Geometry: final body of the model. Coordinates: model frame, mm. A direction names the side the tool comes from. Give positions to 0.01 mm unless a question says otherwise; leave off trailing zeros.
Q1. Reachability of faces 1 (the cylindrical face through (66.487, 109.322, -2.748)), 2 (the cylindrical face through (-97.114, -89.051, 9.903)), 3 (the cylindrical face through (40.74, -98.25, 4.38)) from +Z, -Z, +X, -X, +Y, -Y: full face, straight path, thin tool, end or side. Return the list, or none.
Q2. Pin query (flat end, axial travel): pin 1 Ø3.5 at (x, y) = (63.5, -109.99) entering from -Z; pin 2 Ø1.5 at (y, z) = (26, -4) entering from -X; pin 3 Ø5 at (x, y) = (63.5, 109.99) entering from +Z; pin 4 Ø7 at (x, y) = (-63.5, 109.99) entering from -Z. Return the tip coordinate at first contact, or that it passes through.
Q3. Line query: line 1 (X direction, y = -3.5, z = 8); line 2 (X direction, y = 0, z = 4.25); line 3 (Y direction, x = -63.5, z = -3.5). Output: solid intervals per line, ascending.
Autodesk Inventor part; units mm, degrees
ref_plane "YZ Plane" through (0, 0, 0) normal (1, 0, 0) x (0, 1, 0)
ref_plane "XZ Plane" through (0, 0, 0) normal (0, 1, 0) x (-1, 0, 0)
ref_plane "XY Plane" through (0, 0, 0) normal (0, 0, 1) x (1, 0, 0)
sketch "Sketch1" plane through (0, 0, 0) normal (1, 0, 0) x (0, 1, 0)
  arc A0 (-107.5189, 2.6268) -> (-107.5189, -2.6268) centre (-105.3147, 0) ccw
  line L0 (-105.5687, 3.175) -> (-105.5687, -3.175) construction
  line L1 (-107.5189, 2.6268) -> (-107.5189, 4.635) construction
  line L2 (-106.3625, 5.1846) -> (-106.3625, 3.5971)
  line L3 (-107.5189, 2.6268) -> (-106.3625, 3.5971)
  line L4 (-107.5189, -2.6268) -> (-106.3625, -3.5971)
  line L5 (-134.9375, 5.1846) -> (-134.9375, -6.7721)
  line L6 (-134.9375, 5.1846) -> (-106.3625, 5.1846)
  line L7 (-134.9375, -6.7721) -> (-106.3625, -6.7721)
  line L8 (-106.3625, -6.7721) -> (-106.3625, -3.5971)
  circle A1 centre (-105.5687, 0) radius 3.175 construction
  line L9 (-35.1032, 0) -> (87.3968, 0) construction
  line L10 (-104.775, 5.1846) -> (-104.775, 3.5971) construction
  line L11 (-104.775, -6.7721) -> (-104.775, -3.5971) construction
  line L12 (-103.6186, 2.6268) -> (-104.775, 3.5971) construction
  line L13 (-103.6186, -2.6268) -> (-104.775, -3.5971) construction
  arc A2 (-103.6186, -2.6268) -> (-103.6186, 2.6268) centre (-105.8227, 0) ccw construction
  line L14 (-79.375, 5.1846) -> (-79.375, -6.7721) construction
  line L15 (0, -7.2584) -> (0, 7.2584) construction
  line L16 (-79.375, -6.7721) -> (-104.775, -6.7721) construction
  line L17 (-79.375, 5.1846) -> (-104.775, 5.1846) construction
  line L18 (-104.775, 5.1846) -> (-104.775, 8.3596) construction
  line L19 (-104.775, 8.3596) -> (-79.375, 8.3596) construction
  line L20 (-79.375, 8.3596) -> (-79.375, 5.1846) construction
  line L21 (-90.4875, 22.7342) -> (-90.4875, 8.3596) construction
  point P0 (0, 0)
  point P1 (0, 0)
  point P2 (-108.7437, 0)
  point P3 (-134.9375, -0.7938)
  point P4 (-19.1031, 0)
  point P5 (0, 7.2584)
  point P6 (0, 0)
  point P7 (-119.9381, 21.0485)
  dimension "d0" = 6.35
  dimension "d1" = 3.429
  dimension "d2" = 50
  dimension "d3" = 3.175
  dimension "d4" = 1.5875
  dimension "d5" = 158.75
  dimension "d6" = 3.175
  dimension "d7" = 25.4
  dimension "d8" = 28.575
  dimension "d9" = 180.975
  dimension "d31" = 1.5875
revolve "Revolution1" add sketch "Sketch1" angle 360 about axis through (0, 0, -7.2584) along (0, 0, 1)
sketch "Sketch2" plane through (0, 0, -6.7721) normal (0, 0, 1) x (1, 0, 0)
  point P0 (0, 0)
  point P1 (-127, 0)
  point P2 (-109.9852, -63.5)
  point P3 (-63.5, -109.9852)
  point P4 (0, -127)
  point P5 (63.5, -109.9852)
  point P6 (109.9852, -63.5)
  point P7 (127, 0)
  point P8 (109.9852, 63.5)
  point P9 (63.5, 109.9852)
  point P10 (0, 127)
  point P11 (-63.5, 109.9852)
  point P12 (-109.9852, 63.5)
  dimension "d11" = 127
  dimension "d14" = 360
hole "Hole1" at (-109.9852, -63.5, -6.7721) at (-63.5, -109.9852, -6.7721) at (63.5, -109.9852, -6.7721) at (109.9852, -63.5, -6.7721) at (109.9852, 63.5, -6.7721) at (63.5, 109.9852, -6.7721) at (-63.5, 109.9852, -6.7721) at (-109.9852, 63.5, -6.7721) direction (0, 0, 1) diameter 6.12 depth 7.9375 tip angle 118
sketch "Sketch3" plane through (0, 0, 5.1846) normal (0, 0, 1) x (1, 0, 0)
  circle A0 centre (0, 0) radius 134.9375
  circle A1 centre (0, 0) radius 131.7625
  circle A2 centre (0, 0) radius 134.9375
  dimension "d27" = 3.175
extrude "Extrusion1" add sketch "Sketch3" along normal blind 9.525
fillet "Fillet2" radius 1.5875 3 edges at (-131.7625, 0, 14.7096) (-134.9375, 0, 14.7096) (-131.7625, 0, 5.1846)
properties part number "3DPRINT,TURRET,BEARING,OUTER" material "Nylon 6/6"
Computed:
1. face 1: -Z
1. face 2: +Z
1. face 3: +Z, -Z
2. pin 1: stops at z = 1.95
2. pin 2: stops at x = -132.55
2. pin 3: stops at z = 5.18
2. pin 4: stops at z = -6.77
3. line 1: x = -134.89 to -131.72, 131.72 to 134.89
3. line 2: x = -134.94 to -106.36, 106.36 to 134.94
3. line 3: y = -119.06 to -113.05, -106.93 to -85.47, 85.47 to 106.93, 113.05 to 119.06
